from build123d import *

# Parameters (mm, degrees)
SKETCH1_W           = 152.4
SKETCH1_H           = 101.6
BOSS_EXTRUDE1_DEPTH = 101.6
SKETCH2_W           = 152.4
SKETCH2_H           = 50.8
CUT_EXTRUDE1_DEPTH  = 25.4
SKETCH3_W           = 76.2
SKETCH3_H           = 101.6
CUT_EXTRUDE2_DEPTH  = 25.4
SKETCH4_W           = 76.2
SKETCH4_H           = 101.6
CUT_EXTRUDE3_DEPTH  = 25.4
BOSS_EXTRUDE2_DEPTH = 25.4
SKETCH6_R           = 12.665162167
CUT_EXTRUDE6_DEPTH  = 101.6
SKETCH7_R           = 12.7
CUT_EXTRUDE7_DEPTH  = 50.8
SKETCH8_R           = 19.05
CUT_EXTRUDE8_DEPTH  = 8.382


with BuildPart() as part:
    # Sketch1 → Boss-Extrude1 (new body)
    with BuildSketch(Plane(origin=(0, 0, 0), x_dir=(1, 0, 0), z_dir=(0, 1, 0))):
        with Locations((76.2, 50.8)):
            Rectangle(SKETCH1_W, SKETCH1_H)
    extrude(amount=BOSS_EXTRUDE1_DEPTH)

    # Sketch2 → Cut-Extrude1 (cut)
    with BuildSketch(Plane(origin=(0, 0, 0), x_dir=(-1, 0, 0), z_dir=(0, -1, 0))):
        with Locations((-76.2, 50.8)):
            Rectangle(SKETCH2_W, SKETCH2_H)
    extrude(amount=-CUT_EXTRUDE1_DEPTH, mode=Mode.SUBTRACT)

    # Sketch3 → Cut-Extrude2 (cut)
    with BuildSketch(Plane(origin=(0, 101.6, 0), x_dir=(1, 0, 0), z_dir=(0, 1, 0))):
        with Locations((38.1, 50.8)):
            Rectangle(SKETCH3_W, SKETCH3_H)
    extrude(amount=-CUT_EXTRUDE2_DEPTH, mode=Mode.SUBTRACT)

    # Sketch4 → Cut-Extrude3 (cut)
    with BuildSketch(Plane(origin=(0, 101.6, 0), x_dir=(1, 0, 0), z_dir=(0, 1, 0))):
        with Locations((114.3, 50.8)):
            Rectangle(SKETCH4_W, SKETCH4_H)
    extrude(amount=-CUT_EXTRUDE3_DEPTH, mode=Mode.SUBTRACT)

    # Sketch5 → Boss-Extrude2 (add)
    with BuildSketch(Plane(origin=(0, 76.2, 0), x_dir=(1, 0, 0), z_dir=(0, 1, 0))):
        with BuildLine():
            Line((152.4, 0), (101.6, 0))
            ThreePointArc((101.6, 0), (80.557951031, 50.8), (101.6, 101.6))
            Line((101.6, 101.6), (152.4, 101.6))
            Line((152.4, 101.6), (152.4, 0))
        make_face()
    extrude(amount=BOSS_EXTRUDE2_DEPTH)

    # Sketch6 → Cut-Extrude6 (cut)
    with BuildSketch(Plane(origin=(0, 101.6, 0), x_dir=(1, 0, 0), z_dir=(0, 1, 0))):
        with Locations(Location((114.3, 50.8, 0), (0, 0, 270))):
            Circle(SKETCH6_R)
    extrude(amount=-CUT_EXTRUDE6_DEPTH, mode=Mode.SUBTRACT)

    # Sketch7 → Cut-Extrude7 (cut)
    with BuildSketch(Plane(origin=(0, 76.2, 0), x_dir=(1, 0, 0), z_dir=(0, 1, 0))):
        with Locations(Location((38.1, 50.8, 0), (0, 0, 270))):
            Circle(SKETCH7_R)
    extrude(amount=-CUT_EXTRUDE7_DEPTH, mode=Mode.SUBTRACT)

    # Sketch8 → Cut-Extrude8 (cut)
    with BuildSketch(Plane.XZ.offset(-25.4)):
        with Locations(Location((38.1, -50.8, 0), (0, 0, 270))):
            Circle(SKETCH8_R)
    extrude(amount=-CUT_EXTRUDE8_DEPTH, mode=Mode.SUBTRACT)


solid = part.part
Can you work these out from the model? Positions are in its coordinate system, mm. A direction names the side the tool comes from. Coordinates: 2 decimals unless noted, no trailing zeros. Write each loop counter-clockwise with the first axis right and the second up, starting at its lowest first coordinate (ties: lowest second). Pieces come first, ordered by that corner, then holes. Notation, with made-up numbers: (-6, -14) -> (46, -14) arc R20 ccw to (46, 3) -> close; hole circle Ø4 at (60, 62). An arc over 180 degrees is marked (long way). Write each question's results on one line, items separated by ' | '. Start each with the question number.
Item 1: If we section it at B-B, the plane z = -50.8: Write out the boundary of the cut face in (x, y), and give its area (3 significant figures).
Item 2: Thinking about a two-plate mould opening in X: for faces 1 (the cylindrical face through (48.809, 55.288, -43.973)), 2 (the flat face through (77, 25.4, -51)), 3 (the flat face through (152.4, 50, -52)), which applies, released by +X, released by -X, zero draft, split by the parting line, or undercut?
Item 3: If we section it at C-C, the plane y = 21: Write out the boundary of the cut face in (x, z).
Item 4: I'm going to push flat-ended pins straight in: P1, Ø11.5, axis at x = 45.5, z = -53, coming from the -Y side; P2, Ø3, axis at y = 82.5, z = -89.5, coming from the -X side; P3, Ø6, axis at x = 22, z = -62, coming from the -Y side; P4, Ø23, axis at x = 38.1, z = -50.8, coming from the -Y side. Where does each tip first touch, or does it pass through?
Item 5: On a 3-axis mill with a long thin cutter (end or side, diameter ignored), from which of +Z, -Z, +X, -X, +Y, -Y can I reach the whole of each face in a straight line? I mean faces 4 (the flat face through (34, 33.782, -63)), 5 (the flat face through (77, 13, -76.2)), 6 (the cylindrical face through (80.562, 88.722, -50.01)). Say none if no direction works.
Item 6: If we section it at D-D, the plane x = 114.3: Write out the boundary of the cut face in (y, z).
Item 7: If we section it at A-A, the plane x = 38.1: Write out the boundary of the cut face in (y, z), and give its area (3 significant figures).
Item 8: Please list where these lines run through material, in increasing order: probe 1 along X at (y, z) = (29, -50.8); probe 2 along X at (y, z) = (30, -50); probe 3 along Z at (x, y) = (114, 64).
Answer block:
1) outline: (0, 25.4) -> (19.05, 25.4) -> (19.05, 33.78) -> (25.4, 33.78) -> (25.4, 76.2) -> (0, 76.2) -> close; (50.8, 33.78) -> (57.15, 33.78) -> (57.15, 25.4) -> (101.63, 25.4) -> (101.63, 101.6) -> (80.56, 101.6) -> (80.56, 76.2) -> (50.8, 76.2) -> close; (126.97, 25.4) -> (152.4, 25.4) -> (152.4, 101.6) -> (126.97, 101.6) -> close | area: 6,240 mm²
2) face 1: undercut | face 2: zero draft | face 3: released by +X
3) outline: (0, -101.6) -> (152.4, -101.6) -> (152.4, -76.2) -> (0, -76.2) -> close; (0, -25.4) -> (152.4, -25.4) -> (152.4, 0) -> (0, 0) -> close
4) P1: y = 33.78 | P2: x = 90.94 | P3: y = 25.4 | P4: through
5) face 4: -Y | face 5: +X, -X, -Y | face 6: -X, +Y
6) outline: (0, -101.6) -> (101.6, -101.6) -> (101.6, -63.47) -> (25.4, -63.47) -> (25.4, -76.2) -> (0, -76.2) -> close; (0, -25.4) -> (25.4, -25.4) -> (25.4, -38.13) -> (101.6, -38.13) -> (101.6, 0) -> (0, 0) -> close
7) outline: (0, -101.6) -> (76.2, -101.6) -> (76.2, -63.5) -> (33.78, -63.5) -> (33.78, -69.85) -> (25.4, -69.85) -> (25.4, -76.2) -> (0, -76.2) -> close; (0, -25.4) -> (25.4, -25.4) -> (25.4, -31.75) -> (33.78, -31.75) -> (33.78, -38.1) -> (76.2, -38.1) -> (76.2, 0) -> (0, 0) -> close | area: 5,050 mm²
8) probe 1: 0 to 19.05, 57.15 to 101.63, 126.97 to 152.4 | probe 2: 0 to 19.07, 57.13 to 101.66, 126.94 to 152.4 | probe 3: -101.6 to -63.46, -38.14 to 0
